from build123d import *

# Parameters (mm, degrees)
F0_R     = 1.27
F1_DEPTH = 0.8


with BuildPart() as f1:
    # F0 (on Front) → F1 (new body, symmetric)
    with BuildSketch(Plane.XZ):
        with BuildLine():
            Line((-9.43, -25.4), (9.43, -25.4))
            ThreePointArc((9.43, -25.4), (10.844214, -24.814214), (11.43, -23.4))
            Line((11.43, -23.4), (11.43, 23.4))
            ThreePointArc((11.43, 23.4), (10.844214, 24.814214), (9.43, 25.4))
            Line((9.43, 25.4), (-9.43, 25.4))
            ThreePointArc((-9.43, 25.4), (-10.844214, 24.814214), (-11.43, 23.4))
            Line((-11.43, 23.4), (-11.43, -23.4))
            ThreePointArc((-11.43, -23.4), (-10.844214, -24.814214), (-9.43, -25.4))
        make_face()
        with Locations((-8.89, -22.86)):
            Circle(F0_R, mode=Mode.SUBTRACT)
        with Locations((8.89, -22.86)):
            Circle(F0_R, mode=Mode.SUBTRACT)
        with Locations((-8.89, 22.86)):
            Circle(F0_R, mode=Mode.SUBTRACT)
    extrude(amount=F1_DEPTH, both=True)


solid = f1.part
Build history of the part. All positions in model axes, mm. Round coordinates to 2 decimals unless told otherwise and drop trailing zeros. Loops run counter-clockwise (first coordinate to the right, second up) from the corner with the lowest first, then second, coordinate; pieces in that order, holes last. Notation, with made-up numbers: (86, 38.25) -> (140, 38.25) arc R28 cw to (140, 72.25) -> close; hole circle Ø5 at (13.25, 15). An arc over 180 degrees is marked (long way). Use CSV: the item, a comma, the result in double quotes. Start each with the question number.
Q1. Saw through at D-D on x = -8.89. Give the cut face in (y, z).
Q2. Saw through at C-C on y = -0.2. Give the cut face in (x, z), and give its area (3 significant figures).
Q3. Saw through at B-B on z = -22.86. Give the cut face in (x, y).
Q4. Mould opens along X. For faces 1 (the face through (10.06, 0.01, -23.35)), 2 (the face through (-9.17, 0.01, -24.1)), 3 (the face through (0, -0.8, 0)), 4 (the face through (10.86, -0.01, 24.8)) say: +X half, -X half, draft (parallel to the pull), parting line (faces both ways), or undercut.
Q5. Saw through at A-A on x = 8.89. Give the cut face in (y, z), and give its area (3 significant figures).
Q6. Drill centre lines: L1, parallel to Z at x = -8.89, y = 0.1; L2, parallel to Z at x = 8.89, y = -0.05; L3, parallel to X at y = -0.5, z = -22. Where is each one in solid material? Low to high.
Solutions:
1,outline,"(-0.8, -25.4) -> (0.8, -25.4) -> (0.8, -24.13) -> (-0.8, -24.13) -> close; (-0.8, -21.59) -> (0.8, -21.59) -> (0.8, 21.59) -> (-0.8, 21.59) -> close; (-0.8, 24.13) -> (0.8, 24.13) -> (0.8, 25.4) -> (-0.8, 25.4) -> close"
2,outline,"(-11.43, -23.4) arc R2 ccw to (-9.43, -25.4) -> (9.43, -25.4) arc R2 ccw to (11.43, -23.4) -> (11.43, 23.4) arc R2 ccw to (9.43, 25.4) -> (-9.43, 25.4) arc R2 ccw to (-11.43, 23.4) -> close; hole circle Ø2.54 at (-8.89, -22.86); hole circle Ø2.54 at (-8.89, 22.86); hole circle Ø2.54 at (8.89, -22.86)"
2,area,"1,140 mm^2"
3,outline,"(-11.43, -0.8) -> (-10.16, -0.8) -> (-10.16, 0.8) -> (-11.43, 0.8) -> close; (-7.62, -0.8) -> (7.62, -0.8) -> (7.62, 0.8) -> (-7.62, 0.8) -> close; (10.16, -0.8) -> (11.43, -0.8) -> (11.43, 0.8) -> (10.16, 0.8) -> close"
4,face 1,"undercut"
4,face 2,"undercut"
4,face 3,"draft"
4,face 4,"+X half"
5,outline,"(-0.8, -25.4) -> (0.8, -25.4) -> (0.8, -24.13) -> (-0.8, -24.13) -> close; (-0.8, -21.59) -> (0.8, -21.59) -> (0.8, 25.4) -> (-0.8, 25.4) -> close"
5,area,"77.2 mm^2"
6,L1,"z = -25.4 to -24.13, -21.59 to 21.59, 24.13 to 25.4"
6,L2,"z = -25.4 to -24.13, -21.59 to 25.4"
6,L3,"x = -11.43 to -9.82, -7.96 to 7.96, 9.82 to 11.43"
